```python
from build123d import *

# Parameters (mm, degrees)
F0_W     = 41
F0_H     = 41
F1_DEPTH = 6


with BuildPart() as f1:
    # F0 (on Front) → F1 (new body)
    with BuildSketch(Plane.XZ):
        Polygon((-226.75, -174.116667), (228.25, -174.116667), (248.25, -174.116667), (248.25, -154.116667), (248.25, 150.883333), (248.25, 170.883333), (227.5, 170.883333), (-227.5, 170.883333), (-246.75, 170.883333), (-246.75, 152.5), (-246.75, -152.5), (-246.75, -174.116667), align=None)
        with Locations((-192, -138.116667)):
            Rectangle(F0_W, F0_H, mode=Mode.SUBTRACT)
        with Locations((-121.75, -138.116667)):
            Rectangle(F0_W, F0_H, mode=Mode.SUBTRACT)
        with Locations((-51.5, -138.116667)):
            Rectangle(F0_W, F0_H, mode=Mode.SUBTRACT)
        with Locations((-206.05, -86.616667)):
            Rectangle(F0_W, F0_H, mode=Mode.SUBTRACT)
        with Locations((-149.85, -86.616667)):
            Rectangle(F0_W, F0_H, mode=Mode.SUBTRACT)
        with Locations((-192, -35.116667)):
            Rectangle(F0_W, F0_H, mode=Mode.SUBTRACT)
        with Locations((-93.65, -86.616667)):
            Rectangle(F0_W, F0_H, mode=Mode.SUBTRACT)
        with Locations((-37.45, -86.616667)):
            Rectangle(F0_W, F0_H, mode=Mode.SUBTRACT)
        with Locations((-121.75, -35.116667)):
            Rectangle(F0_W, F0_H, mode=Mode.SUBTRACT)
        with Locations((-51.5, -35.116667)):
            Rectangle(F0_W, F0_H, mode=Mode.SUBTRACT)
        with Locations((53, -138.116667)):
            Rectangle(F0_W, F0_H, mode=Mode.SUBTRACT)
        with Locations((123.25, -138.116667)):
            Rectangle(F0_W, F0_H, mode=Mode.SUBTRACT)
        with Locations((193.5, -138.116667)):
            Rectangle(F0_W, F0_H, mode=Mode.SUBTRACT)
        with Locations((38.95, -86.616667)):
            Rectangle(F0_W, F0_H, mode=Mode.SUBTRACT)
        with Locations((95.15, -86.616667)):
            Rectangle(F0_W, F0_H, mode=Mode.SUBTRACT)
        with Locations((53, -35.116667)):
            Rectangle(F0_W, F0_H, mode=Mode.SUBTRACT)
        with Locations((123.25, -35.116667)):
            Rectangle(F0_W, F0_H, mode=Mode.SUBTRACT)
        with Locations((151.35, -86.616667)):
            Rectangle(F0_W, F0_H, mode=Mode.SUBTRACT)
        with Locations((207.55, -86.616667)):
            Rectangle(F0_W, F0_H, mode=Mode.SUBTRACT)
        with Locations((193.5, -35.116667)):
            Rectangle(F0_W, F0_H, mode=Mode.SUBTRACT)
        with Locations((-192, 31.883333)):
            Rectangle(F0_W, F0_H, mode=Mode.SUBTRACT)
        with Locations((-206.05, 83.383333)):
            Rectangle(F0_W, F0_H, mode=Mode.SUBTRACT)
        with Locations((-149.85, 83.383333)):
            Rectangle(F0_W, F0_H, mode=Mode.SUBTRACT)
        with Locations((-121.75, 31.883333)):
            Rectangle(F0_W, F0_H, mode=Mode.SUBTRACT)
        with Locations((-51.5, 31.883333)):
            Rectangle(F0_W, F0_H, mode=Mode.SUBTRACT)
        with Locations((-93.65, 83.383333)):
            Rectangle(F0_W, F0_H, mode=Mode.SUBTRACT)
        with Locations((-37.45, 83.383333)):
            Rectangle(F0_W, F0_H, mode=Mode.SUBTRACT)
        with Locations((-192, 134.883333)):
            Rectangle(F0_W, F0_H, mode=Mode.SUBTRACT)
        with Locations((-121.75, 134.883333)):
            Rectangle(F0_W, F0_H, mode=Mode.SUBTRACT)
        with Locations((-51.5, 134.883333)):
            Rectangle(F0_W, F0_H, mode=Mode.SUBTRACT)
        with Locations((53, 31.883333)):
            Rectangle(F0_W, F0_H, mode=Mode.SUBTRACT)
        with Locations((123.25, 31.883333)):
            Rectangle(F0_W, F0_H, mode=Mode.SUBTRACT)
        with Locations((38.95, 83.383333)):
            Rectangle(F0_W, F0_H, mode=Mode.SUBTRACT)
        with Locations((95.15, 83.383333)):
            Rectangle(F0_W, F0_H, mode=Mode.SUBTRACT)
        with Locations((193.5, 31.883333)):
            Rectangle(F0_W, F0_H, mode=Mode.SUBTRACT)
        with Locations((151.35, 83.383333)):
            Rectangle(F0_W, F0_H, mode=Mode.SUBTRACT)
        with Locations((207.55, 83.383333)):
            Rectangle(F0_W, F0_H, mode=Mode.SUBTRACT)
        with Locations((53, 134.883333)):
            Rectangle(F0_W, F0_H, mode=Mode.SUBTRACT)
        with Locations((123.25, 134.883333)):
            Rectangle(F0_W, F0_H, mode=Mode.SUBTRACT)
        with Locations((193.5, 134.883333)):
            Rectangle(F0_W, F0_H, mode=Mode.SUBTRACT)
    extrude(amount=F1_DEPTH)


solid = f1.part
```
The listing builds one solid part. Answer for the finished solid, in the listing's coordinates (mm). Give positions to 0.01 mm unless a question says otherwise; leave off trailing zeros. Loops run counter-clockwise (first coordinate to the right, second up) from the corner with the lowest first, then second, coordinate; pieces in that order, holes last. Notation, with made-up numbers: (53.5, -13) - (109.5, -13) arc R31 ccw to (109.5, 17) - close; hole circle Ø5 at (47, 19.5). An arc over 180 degrees is marked (long way). Return JSON: item names as keys, results as strings. Group by question number.
1. Find section D-D (x = -177). Write down the section's boundary in (y, z), then the cut area to 3 significant figures.
2. Find section A-A (x = 94.5). Write down the section's boundary in (y, z).
3. Straight lines are drawn through the part: line 1 (Z direction, x = -181.5, y = -1.85); line 2 (Z direction, x = -82, y = -4.6). For each, find the intervals that lie inside material, in ascending order. Write a range as [from, to].
4. Find section B-B (z = 122.5). Write down the section's boundary in (x, y).
5. Find section C-C (x = 201). Write down the section's boundary in (y, z).
Verdict:
{
 "1": {"outline": "(-6, -174.12) - (0, -174.12) - (0, -158.62) - (-6, -158.62) - close; (-6, -117.62) - (0, -117.62) - (0, -55.62) - (-6, -55.62) - close; (-6, -14.62) - (0, -14.62) - (0, 11.38) - (-6, 11.38) - close; (-6, 52.38) - (0, 52.38) - (0, 114.38) - (-6, 114.38) - close; (-6, 155.38) - (0, 155.38) - (0, 170.88) - (-6, 170.88) - close", "area": "1,090 mm^2"},
 "2": {"outline": "(-6, -174.12) - (0, -174.12) - (0, -107.12) - (-6, -107.12) - close; (-6, -66.12) - (0, -66.12) - (0, 62.88) - (-6, 62.88) - close; (-6, 103.88) - (0, 103.88) - (0, 170.88) - (-6, 170.88) - close"},
 "3": {"line 1": "z = [-174.12, -158.62], [-117.62, -55.62], [-14.62, 11.38], [52.38, 114.38], [155.38, 170.88]", "line 2": "z = [-174.12, -107.12], [-66.12, 62.88], [103.88, 170.88]"},
 "4": {"outline": "(-246.75, -6) - (-212.5, -6) - (-212.5, 0) - (-246.75, 0) - close; (-171.5, -6) - (-142.25, -6) - (-142.25, 0) - (-171.5, 0) - close; (-101.25, -6) - (-72, -6) - (-72, 0) - (-101.25, 0) - close; (-31, -6) - (32.5, -6) - (32.5, 0) - (-31, 0) - close; (73.5, -6) - (102.75, -6) - (102.75, 0) - (73.5, 0) - close; (143.75, -6) - (173, -6) - (173, 0) - (143.75, 0) - close; (214, -6) - (248.25, -6) - (248.25, 0) - (214, 0) - close"},
 "5": {"outline": "(-6, -174.12) - (0, -174.12) - (0, -158.62) - (-6, -158.62) - close; (-6, -117.62) - (0, -117.62) - (0, -107.12) - (-6, -107.12) - close; (-6, -66.12) - (0, -66.12) - (0, -55.62) - (-6, -55.62) - close; (-6, -14.62) - (0, -14.62) - (0, 11.38) - (-6, 11.38) - close; (-6, 52.38) - (0, 52.38) - (0, 62.88) - (-6, 62.88) - close; (-6, 103.88) - (0, 103.88) - (0, 114.38) - (-6, 114.38) - close; (-6, 155.38) - (0, 155.38) - (0, 170.88) - (-6, 170.88) - close"}
}
